Source: CAD feature listing. Evaluate the final solid. Frame: model axes, mm. Face numbers are marked on the shaded views. A direction names the side the tool comes from. Give positions to 0.01 mm unless a question says otherwise; leave off trailing zeros. Order: outer loops, then holes, each group sorted by start corner. A loop starts at its lowest first (then second) coordinate and runs counter-clockwise, first axis right, second up.
```python
from build123d import *

# Parameters (mm, degrees)
F1_DEPTH = 30
F2_R     = 11
F3_DEPTH = 0.5
F4_T     = -2.5
F5_R     = 11
F6_DEPTH = 1
F7_R     = 5
F8_DEPTH = 1.5
F9_SIZE2 = 4
F9_SIZE  = 4


with BuildPart() as f1:
    # F0 (on Front) → F1 (new body)
    with BuildSketch(Plane.XZ):
        Polygon((42.5, -55), (42.5, 55), (-24.856195, 55), (-42.5, 37.632745), (-42.5, -55), align=None)
        Polygon((-42.5, 37.632745), (-24.856195, 55), (-42.5, 55), align=None)
    extrude(amount=F1_DEPTH)

    # F2 (on face) → F3 (join)
    with BuildSketch(Plane.XY.offset(55)):
        with Locations((25.320798, -14.402656)):
            Circle(F2_R)
    extrude(amount=-F3_DEPTH)

    # F4
    f4_openings = [f1.faces().sort_by_distance(p)[0] for p in [
        (0, -30, 0),
    ]]
    offset(amount=F4_T, openings=f4_openings)

    # F5 (on face) → F6 (cut)
    with BuildSketch(Plane.XY.offset(55)):
        with Locations((27.876107, -15.56416)):
            Circle(F5_R)
    extrude(amount=-F6_DEPTH, mode=Mode.SUBTRACT)

    # F7 (on face) → F8 (cut)
    with BuildSketch(Plane.XY.offset(54)):
        with Locations((27.876107, -15.56416)):
            Circle(F7_R)
    extrude(amount=-F8_DEPTH, mode=Mode.SUBTRACT)

    # F9
    f9_edges = [f1.edges().sort_by_distance(p)[0] for p in [
        (-42.5, -15, 55),
    ]]
    chamfer(f9_edges, length=F9_SIZE, length2=F9_SIZE2)


solid = f1.part
```
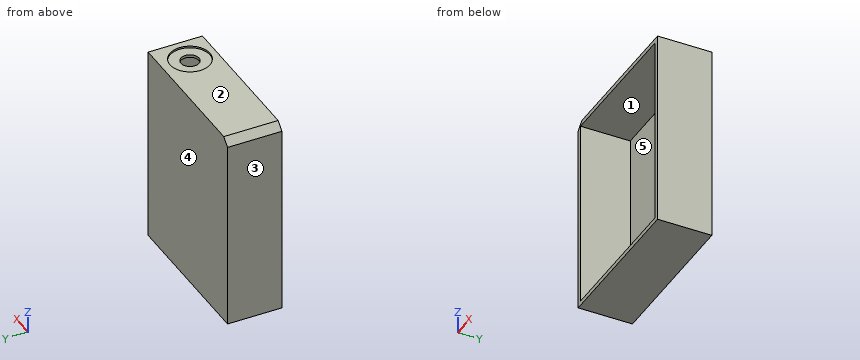
1) Section query A-A, the plane x = 29. Return the cut outline in (y, z), and give its area (3 significant figures).
Report:
outline: (-30, -55) - (0, -55) - (0, 55) - (-4.62, 55) - (-4.62, 54) - (-10.69, 54) - (-10.69, 52.5) - (-2.5, 52.5) - (-2.5, -52.5) - (-30, -52.5) - close; (-30, 52.5) - (-20.44, 52.5) - (-20.44, 54) - (-26.51, 54) - (-26.51, 55) - (-30, 55) - close
area: 376 mm2
2) Draft query along X for the marked faces 3, 4 and 5. Return one class per face: +X half, -X half, draft (parallel to the pull), parting line (faces both ways), or undercut.
Report:
face 3: -X half
face 4: draft
face 5: undercut
3) Section query D-D, the plane y = -17. Return the cut outline in (x, z).
Report:
outline: (-42.5, -55) - (42.5, -55) - (42.5, 55) - (38.78, 55) - (38.78, 54) - (32.67, 54) - (32.67, 52.5) - (40, 52.5) - (40, -52.5) - (-40, -52.5) - (-40, 52.5) - (23.09, 52.5) - (23.09, 54) - (16.97, 54) - (16.97, 55) - (-38.5, 55) - (-42.5, 51) - close
4) Reachability of the marked faces 1 and 2 from +Z, -Z, +X, -X, +Y, -Y: full face, straight path, thin tool, end or side. Return the list, or none.
Report:
face 1: -Y
face 2: +Z, +X, -X, +Y, -Y
5) Section query B-B, the plane z = -13. Return the cut outline in (x, y), and give its area (3 significant figures).
Report:
outline: (-42.5, -30) - (-40, -30) - (-40, -2.5) - (40, -2.5) - (40, -30) - (42.5, -30) - (42.5, 0) - (-42.5, 0) - close
area: 350 mm2
6) Pin query (flat end, axial travel): pin 1 (10 mm diameter, centred on x = 21, z = -15.5, fed in from +Y); pin 2 (1.5 mm diameter, centred on x = -15, z = 34, fed in from -Y); pin 3 (6 mm diameter, centred on x = 27.88, y = -15.56, fed in from +Z). Return the tip coordinate at first contact, or that it passes through.
Report:
pin 1: stops at y = 0
pin 2: stops at y = -2.5
pin 3: stops at z = -52.5
7) Material intervals for L1, parallel to Z at x = -24.5, y = -20; L2, parallel to X at y = -16.5, z = -16; L3, parallel to Y at x = 34, z = -39, sorted ascending.
Report:
L1: z = -55 to -52.5, 52.5 to 55
L2: x = -42.5 to -40, 40 to 42.5
L3: y = -2.5 to 0
8) Section query C-C, the plane x = 15. Return the cut outline in (y, z).
Report:
outline: (-30, -55) - (0, -55) - (0, 55) - (-30, 55) - (-30, 52.5) - (-2.5, 52.5) - (-2.5, -52.5) - (-30, -52.5) - close
